Geometry check sheet. Reference: the model listing, model coordinates, mm. A direction names the side the tool comes from. Round coordinates to 2 decimals unless told otherwise and drop trailing zeros. Loops run counter-clockwise (first coordinate to the right, second up) from the corner with the lowest first, then second, coordinate; pieces in that order, holes last. Notation, with made-up numbers: (-13, 58) -> (23, 58) arc R35 cw to (23, 94) -> close; hole circle Ø2 at (-36, 17.25). An arc over 180 degrees is marked (long way). Use one line per item in the form item = value.
from build123d import *

# Parameters (mm, degrees)
F0_W     = 134
F0_H     = 3
F0_W_2   = 36
F0_H_2   = 4
F0_R     = 3.75
F1_DEPTH = 4
F2_DEPTH = 26
F3_DEPTH = 12
F4_R     = 3.99999


# Not quite as in the source:
# - a fillet or chamfer is up to 0.001 mm smaller than in the source, because OpenCascade refuses the exact size


with BuildPart() as f1:
    # F0 (on Top) → F1 (new body)
    with BuildSketch(Plane.XY):
        with Locations((67, -1.5)):
            Rectangle(F0_W, F0_H)
        with Locations((22, -83)):
            Rectangle(F0_W_2, F0_H_2)
        Polygon((134, -3), (0, -3), (0, -85), (4, -85), (4, -81), (40, -81), (40, -85), (134, -85), align=None)
        with Locations((120, -60)):
            Circle(F0_R, mode=Mode.SUBTRACT)
        with Locations((120, -25)):
            Circle(F0_R, mode=Mode.SUBTRACT)
    extrude(amount=F1_DEPTH)

    # F0 (on Top) → F2 (join)
    with BuildSketch(Plane.XY):
        with Locations((67, -1.5)):
            Rectangle(F0_W, F0_H)
    extrude(amount=F2_DEPTH)

    # F0 (on Top) → F3 (join)
    with BuildSketch(Plane.XY):
        with Locations((22, -83)):
            Rectangle(F0_W_2, F0_H_2)
    extrude(amount=F3_DEPTH)

    # F4 (radius 4 in the source; OpenCascade refuses exactly that, so slightly less here)
    f4_edges = [f1.edges().sort_by_distance(p)[0] for p in [
        (67, -85, 0),
        (134, -42.5, 0),
        (0, -42.5, 0),
        (67, 0, 0),
        (134, 0, 13),
        (0, 0, 13),
        (134, -85, 2),
        (0, -85, 2),
    ]]
    fillet(f4_edges, radius=F4_R)


solid = f1.part
1. Gauge pin test, flat ends, axial feed: pin 1 (4.5 mm diameter, centred on x = 120, y = -25, fed in from -Z); pin 2 (2 mm diameter, centred on y = -82.5, z = 7.5, fed in from -X); pin 3 (4.5 mm diameter, centred on y = -83, z = 8, fed in from +X); pin 4 (4.5 mm diameter, centred on x = 28.5, y = -82.5, fed in from +Z). Record the tip position at first contact, or that the pin passes through.
Return value:
pin_1 = through
pin_2 = 4
pin_3 = 40
pin_4 = 12
2. Tool access check on faces 1 (the flat face through (40, -83, 8)), 2 (the flat face through (4, -83, 8)), 3 (the flat face through (22, -81, 8)). Record the directions out of +Z, -Z, +X, -X, +Y, -Y that give a thin tool (end or side, any length) a straight path to the whole face; none if there is none.
Return value:
face_1 = +Z, +X, -Y
face_2 = +Z, -X, -Y
face_3 = +Z, +X, -X
3. Material ranges on line 1 along Y through (x, z) = (120, 3); line 2 along Y through (x, z) = (120, 1.65); line 3 along Y through (x, z) = (115, 8), recorded low to high.
Return value:
line_1 = -84.87 to -63.75, -56.25 to -28.75, -21.25 to -0.13
line_2 = -84.24 to -63.75, -56.25 to -28.75, -21.25 to -0.76
line_3 = -3 to 0
4. Section check B-B (x = 120). Count the separate pieces of the cut face and the enclosed holes in it, then the cut area to 3 significant figures.
Return value:
separate_pieces = 3
enclosed_holes = 0
area = 339 mm2
5. Section check D-D (x = 38.5). Record the boundary of the cut face in (y, z), then the cut area to 3 significant figures.
Return value:
outline = (-85, 4) arc R4 ccw to (-81, 0) -> (-4, 0) arc R4 ccw to (0, 4) -> (0, 26) -> (-3, 26) -> (-3, 4) -> (-81, 4) -> (-81, 12) -> (-85, 12) -> close
area = 431 mm2
6. Section check C-C (z = 6). Record the boundary of the cut face in (x, y).
Return value:
outline = (0.13, -3) -> (133.87, -3) arc R4 ccw to (130, 0) -> (4, 0) arc R4 ccw to start; (4, -85) -> (40, -85) -> (40, -81) -> (4, -81) -> close
